Job drawing, mm, ordinate dimensions from the low corner. One solid piece. Give positions to 0.01 mm unless a question says otherwise; leave off trailing zeros. Loops run counter-clockwise (first coordinate to the right, second up) from the corner with the lowest first, then second, coordinate; pieces in that order, holes last. Notation, with made-up numbers: (-31, 43) - (0, 43) arc R16 ccw to (0, 66) - close; hole circle Ø7 at (0.5, 84.25). An arc over 180 degrees is marked (long way). Use a Markdown table: item, result.
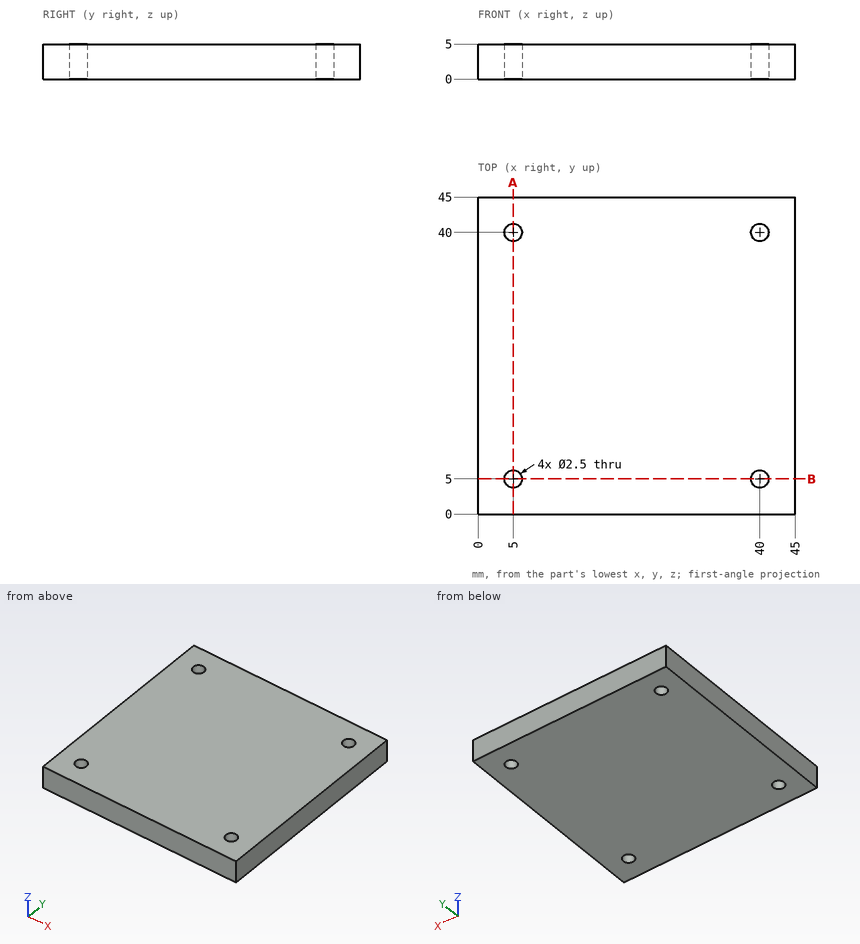
(1) Pin check, flat tip, straight feed: P1, Ø2, axis at y = 21, z = 2, coming from the -X side. Stop position of the tip, or through.
Computed:
| item | result |
|---|---|
| P1 | x = 0 |
(2) Slice it at A-A, the plane x = 5. Write the cut outline in (y, z), plus the area to 3 significant figures.
Computed:
| item | result |
|---|---|
| outline | (0, 0) - (3.75, 0) - (3.75, 5) - (0, 5) - close; (6.25, 0) - (38.75, 0) - (38.75, 5) - (6.25, 5) - close; (41.25, 0) - (45, 0) - (45, 5) - (41.25, 5) - close |
| area | 200 mm² |
(3) Drill centre lines: probe 1 along Y at (x, z) = (40, 3.55); probe 2 along X at (y, z) = (5.5, 0.95); probe 3 along Y at (x, z) = (39, 2.2). Where is each one in solid material? Low to high. Write a range as [from, to].
Computed:
| item | result |
|---|---|
| probe 1 | [0, 3.75], [6.25, 38.75], [41.25, 45] |
| probe 2 | [0, 3.85], [6.15, 38.85], [41.15, 45] |
| probe 3 | [0, 4.25], [5.75, 39.25], [40.75, 45] |
